Can you work these out from the drawing? Everything is in mm from the part's minimum corner. A direction names the side the tool comes from. Coordinates: 2 decimals unless noted, no trailing zeros. Loops run counter-clockwise (first coordinate to the right, second up) from the corner with the lowest first, then second, coordinate; pieces in that order, holes last. Notation, with made-up numbers: (48.25, 52) -> (79.25, 52) arc R14 ccw to (79.25, 58) -> close; hole circle Ø5 at (-18.75, 86). An arc over 180 degrees is marked (long way). Put each result on its own line as item: value. Start each with the question number.
Item 1: If we section it at B-B on x = 1088: Please give me the cut outline in (y, z).
Item 2: If we section it at A-A on z = 512: Please give me the cut outline in (x, y), plus the area to 3 significant figures.
Item 3: If we section it at D-D on z = 179: Please give me the cut outline in (x, y) (1 decimal).
Item 4: We'd pull the mould along X, two halves only. Please class the marked faces 3, 4 and 5: pulls with the +X half, pulls with the -X half, needs draft (parallel to the pull), parting line crosses it, or undercut.
Item 5: For the marked faces 1 and 2, which set-ups out of +Z, -Z, +X, -X, +Y, -Y let a thin tool reach every point of the face, with its end or its side?
Item 6: If we section it at C-C on y = 540: Please give me the cut outline in (x, z).
Item 7: Please list where these lines run through material, in increasing order: L1, parallel to X at y = 591.5, z = 357.5; L2, parallel to Y at x = 1859, z = 603; L3, parallel to Y at x = 163, z = 445. Write a range as from..to.
Item 8: Will these pins go through, and if not, where does the flat tip stop? P1, Ø10, axis at y = 542, z = 171.5, coming from the -X side; P2, Ø22.5, axis at x = 2048, z = 32, coming from the +Y side; P3, Ø22.5, axis at y = 66.5, z = 424, coming from the -X side.
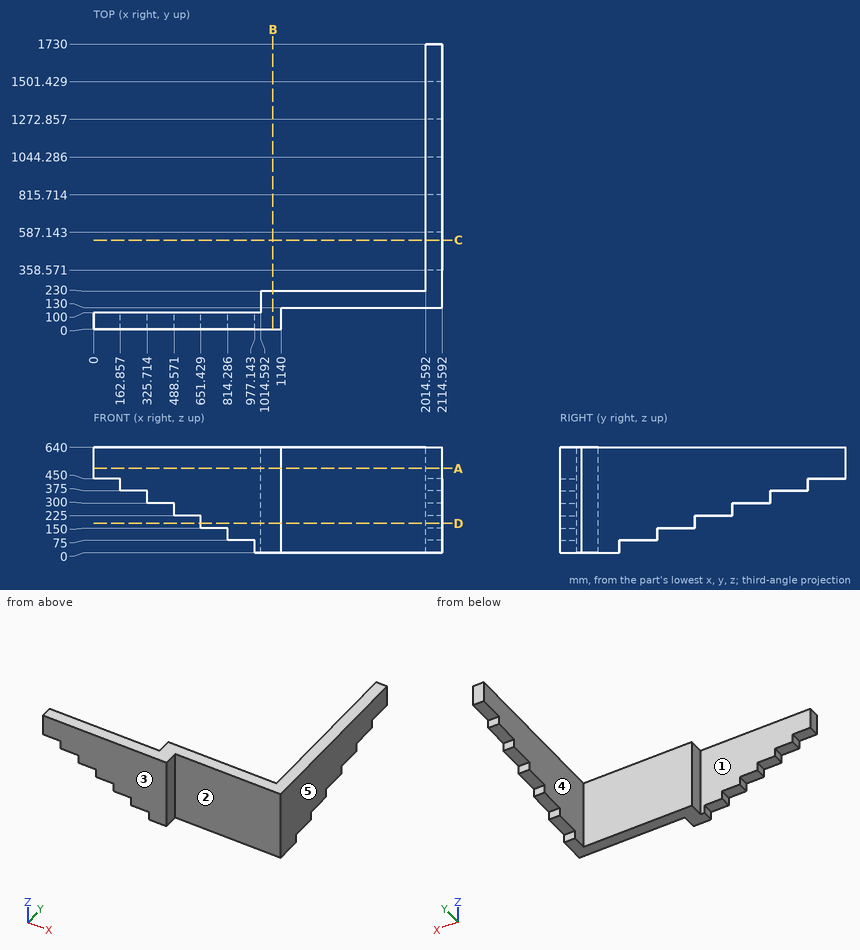
Solutions:
1. outline: (0, 0) -> (230, 0) -> (230, 640) -> (0, 640) -> close
2. outline: (0, 0) -> (1140, 0) -> (1140, 130) -> (2114.59, 130) -> (2114.59, 1730) -> (2014.59, 1730) -> (2014.59, 230) -> (1014.59, 230) -> (1014.59, 100) -> (0, 100) -> close
2. area: 378,000 mm^2
3. outline: (651.4, 0) -> (1140, 0) -> (1140, 130) -> (2114.6, 130) -> (2114.6, 815.7) -> (2014.6, 815.7) -> (2014.6, 230) -> (1014.6, 230) -> (1014.6, 100) -> (651.4, 100) -> close
4. face 3: needs draft
4. face 4: pulls with the -X half
4. face 5: pulls with the +X half
5. face 1: +Z, -Z, -X, +Y
5. face 2: +Z, -Z, +X, -Y
6. outline: (2014.59, 75) -> (2114.59, 75) -> (2114.59, 640) -> (2014.59, 640) -> close
7. L1: 2014.59..2114.59
7. L2: 130..230
7. L3: 0..100
8. P1: x = 2014.59
8. P2: y = 358.57
8. P3: x = 162.86
